from build123d import *

# Parameters (mm, degrees)
BOSS_EXTRUDE1_DEPTH = 5
FILLET1_R           = 8
SKETCH2_R           = 10
SKETCH2_R_2         = 3.1
CUT_EXTRUDE1_DEPTH  = 10


with BuildPart() as part:
    # Sketch1 → Boss-Extrude1 (new body)
    with BuildSketch(Plane(origin=(0, 0, 0), x_dir=(1, 0, 0), z_dir=(0, 1, 0))):
        Polygon((-57.735026919, 0), (-28.867513459, -50), (28.867513459, -50), (57.735026919, 0), (28.867513459, 50), (-28.867513459, 50), align=None)
    extrude(amount=BOSS_EXTRUDE1_DEPTH)

    # Fillet1
    fillet1_edges = [part.edges().sort_by_distance(p)[0] for p in [
        (-28.867513459, 2.5, -50),
        (28.867513459, 2.5, -50),
        (57.735026919, 2.5, 0),
        (28.867513459, 2.5, 50),
        (-28.867513459, 2.5, 50),
        (-57.735026919, 2.5, 0),
    ]]
    fillet(fillet1_edges, radius=FILLET1_R)

    # Sketch2 → Cut-Extrude1 (cut)
    with BuildSketch(Plane(origin=(0, 5, 0), x_dir=(1, 0, 0), z_dir=(0, 1, 0))):
        with Locations(Location((0, 0, 0), (0, 0, 270))):
            Circle(SKETCH2_R)
        with Locations(Location((-25.5, 44.167295593, 0), (0, 0, 270))):
            Circle(SKETCH2_R_2)
        with Locations(Location((25.5, 44.167295593, 0), (0, 0, 270))):
            Circle(SKETCH2_R_2)
        with Locations(Location((51, 0, 0), (0, 0, 270))):
            Circle(SKETCH2_R_2)
        with Locations(Location((25.5, -44.167295593, 0), (0, 0, 270))):
            Circle(SKETCH2_R_2)
        with Locations(Location((-25.5, -44.167295593, 0), (0, 0, 270))):
            Circle(SKETCH2_R_2)
        with Locations(Location((-51, 0, 0), (0, 0, 270))):
            Circle(SKETCH2_R_2)
        with BuildLine():
            Line((6.206515394, 20.75), (16.454482672, 38.5))
            ThreePointArc((16.454482672, 38.5), (16.454482672, 39.5), (15.588457268, 40))
            Line((15.588457268, 40), (-15.588457268, 40))
            ThreePointArc((-15.588457268, 40), (-16.454482672, 39.5), (-16.454482672, 38.5))
            Line((-16.454482672, 38.5), (-6.206515394, 20.75))
            ThreePointArc((-6.206515394, 20.75), (-5.657477288, 20.200961894), (-4.907477288, 20))
            Line((-4.907477288, 20), (4.907477288, 20))
            ThreePointArc((4.907477288, 20), (5.657477288, 20.200961894), (6.206515394, 20.75))
        make_face()
        with BuildLine():
            Line((21.073284825, 5), (41.569219382, 5))
            ThreePointArc((41.569219382, 5), (42.435244785, 5.5), (42.435244785, 6.5))
            Line((42.435244785, 6.5), (26.846787517, 33.5))
            ThreePointArc((26.846787517, 33.5), (25.980762114, 34), (25.11473671, 33.5))
            Line((25.11473671, 33.5), (14.866769432, 15.75))
            ThreePointArc((14.866769432, 15.75), (14.665807537, 15), (14.866769432, 14.25))
            Line((14.866769432, 14.25), (19.77424672, 5.75))
            ThreePointArc((19.77424672, 5.75), (20.323284825, 5.200961894), (21.073284825, 5))
        make_face()
        with BuildLine():
            Line((14.866769432, -15.75), (25.11473671, -33.5))
            ThreePointArc((25.11473671, -33.5), (25.980762114, -34), (26.846787517, -33.5))
            Line((26.846787517, -33.5), (42.435244785, -6.5))
            ThreePointArc((42.435244785, -6.5), (42.435244785, -5.5), (41.569219382, -5))
            Line((41.569219382, -5), (21.073284825, -5))
            ThreePointArc((21.073284825, -5), (20.323284825, -5.200961894), (19.77424672, -5.75))
            Line((19.77424672, -5.75), (14.866769432, -14.25))
            ThreePointArc((14.866769432, -14.25), (14.665807537, -15), (14.866769432, -15.75))
        make_face()
        with BuildLine():
            Line((-21.073284825, -5), (-41.569219382, -5))
            ThreePointArc((-41.569219382, -5), (-42.435244785, -5.5), (-42.435244785, -6.5))
            Line((-42.435244785, -6.5), (-26.846787517, -33.5))
            ThreePointArc((-26.846787517, -33.5), (-25.980762114, -34), (-25.11473671, -33.5))
            Line((-25.11473671, -33.5), (-14.866769432, -15.75))
            ThreePointArc((-14.866769432, -15.75), (-14.665807537, -15), (-14.866769432, -14.25))
            Line((-14.866769432, -14.25), (-19.77424672, -5.75))
            ThreePointArc((-19.77424672, -5.75), (-20.323284825, -5.200961894), (-21.073284825, -5))
        make_face()
        with BuildLine():
            Line((-14.866769432, 15.75), (-25.11473671, 33.5))
            ThreePointArc((-25.11473671, 33.5), (-25.980762114, 34), (-26.846787517, 33.5))
            Line((-26.846787517, 33.5), (-42.435244785, 6.5))
            ThreePointArc((-42.435244785, 6.5), (-42.435244785, 5.5), (-41.569219382, 5))
            Line((-41.569219382, 5), (-21.073284825, 5))
            ThreePointArc((-21.073284825, 5), (-20.323284825, 5.200961894), (-19.77424672, 5.75))
            Line((-19.77424672, 5.75), (-14.866769432, 14.25))
            ThreePointArc((-14.866769432, 14.25), (-14.665807537, 15), (-14.866769432, 15.75))
        make_face()
    extrude(amount=-CUT_EXTRUDE1_DEPTH, mode=Mode.SUBTRACT)


solid = part.part
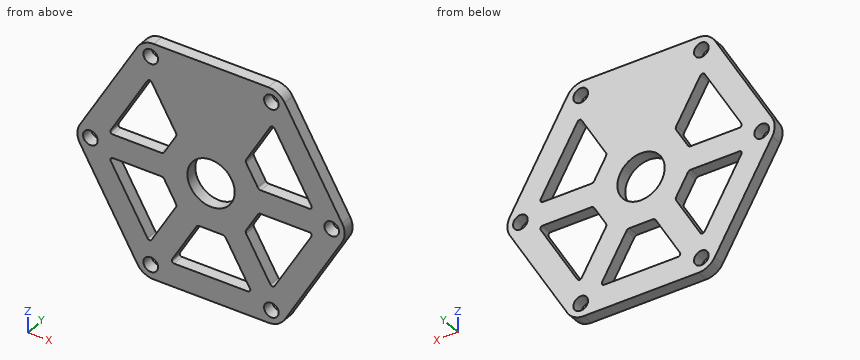
Could you check a few things on this model? Use its own coordinates, in mm. Give positions to 0.01 mm unless a question says otherwise; leave off trailing zeros. Write each loop counter-clockwise with the first axis right and the second up, starting at its lowest first coordinate (ties: lowest second). Pieces come first, ordered by that corner, then holes. Notation, with made-up numbers: (46, -6.75) -> (55, -6.75) arc R24 ccw to (55, 15.25) -> close; hole circle Ø9 at (-36, -8.5). An arc over 180 degrees is marked (long way). Answer as CSV lines item,"result". Start each with the question number.
(1) If we section it at A-A, the plane z = 0: Write out the boundary of the cut face in (x, y).
(2) If we section it at D-D, the plane x = 51: Write out the boundary of the cut face in (y, z).
(3) If we section it at B-B, the plane x = 0: Write out the boundary of the cut face in (y, z).
(4) I'm going to push flat-ended pins straight in: pin 1 Ø12 at (x, z) = (0, 0) entering from -Y; pin 2 Ø1.5 at (x, y) = (-30.5, 3.5) entering from +Z; pin 3 Ø2.5 at (x, y) = (34.5, 3) entering from -Z; pin 4 Ø1.5 at (y, z) = (3, -34.5) entering from +X. Where does each tip first touch, or does it pass through?
(5) If we section it at C-C, the plane y = 2.35: Give the number of separate pieces and of enclosed holes in the cut face, and give its area (3 significant figures).
(6) Please list where these lines run through material, in increasing order: line 1 (X direction, y = 2.1, z = 0); line 2 (X direction, y = 1.6, z = 31.5); line 3 (X direction, y = 2.95, z = -1.5).
Answer list:
1,outline,"(-56.5, 0) -> (-54.1, 0) -> (-54.1, 5) -> (-56.5, 5) -> close; (-47.9, 0) -> (-10, 0) -> (-10, 5) -> (-47.9, 5) -> close; (10, 0) -> (47.9, 0) -> (47.9, 5) -> (10, 5) -> close; (54.1, 0) -> (56.5, 0) -> (56.5, 5) -> (54.1, 5) -> close"
2,outline,"(0, -11.67) -> (5, -11.67) -> (5, -3.1) -> (0, -3.1) -> close; (0, 3.1) -> (5, 3.1) -> (5, 11.67) -> (0, 11.67) -> close"
3,outline,"(0, -50) -> (5, -50) -> (5, -40) -> (0, -40) -> close; (0, -20) -> (5, -20) -> (5, -10) -> (0, -10) -> close; (0, 10) -> (5, 10) -> (5, 50) -> (0, 50) -> close"
4,pin 1,"through"
4,pin 2,"z = 47.81"
4,pin 3,"z = -42.41"
4,pin 4,"x = 38.25"
5,separate pieces,"1"
5,enclosed holes,"12"
5,area,"5,840 mm^2"
6,line 1,"-56.5 to -54.1, -47.9 to -10, 10 to 47.9, 54.1 to 56.5"
6,line 2,"-39.55 to -28, -23.96 to 23.96, 28 to 39.55"
6,line 3,"-56.36 to -53.71, -48.29 to -9.89, 9.89 to 48.29, 53.71 to 56.36"
